from build123d import *

# Parameters (mm, degrees)
SKETCH2_W           = 43.5
SKETCH2_H           = 43.5
BOSS_EXTRUDE1_DEPTH = 5
SKETCH4_W           = 23
SKETCH4_H           = 16
BOSS_EXTRUDE2_DEPTH = 26
SKETCH5_W           = 6
SKETCH5_H           = 10
SKETCH5_W_2         = 12
SKETCH5_H_2         = 6
BOSS_EXTRUDE3_DEPTH = 10
SKETCH6_R           = 2.5
CUT_EXTRUDE1_DEPTH  = 41.275612969


with BuildPart() as part:
    # Sketch2 → Boss-Extrude1 (new body)
    with BuildSketch(Plane(origin=(0, 0, 0), x_dir=(1, 0, 0), z_dir=(0, 1, 0))):
        Rectangle(SKETCH2_W, SKETCH2_H)
    extrude(amount=BOSS_EXTRUDE1_DEPTH)

    # Sketch4 → Boss-Extrude2 (add)
    with BuildSketch(Plane(origin=(0, 5, 0), x_dir=(1, 0, 0), z_dir=(0, 1, 0))):
        with Locations((0, -13.75)):
            Rectangle(SKETCH4_W, SKETCH4_H)
    extrude(amount=BOSS_EXTRUDE2_DEPTH)

    # Sketch5 → Boss-Extrude3 (add)
    with BuildSketch(Plane(origin=(0, 5, 0), x_dir=(1, 0, 0), z_dir=(0, 1, 0))):
        with Locations((-18.75, 9.331650707)):
            Rectangle(SKETCH5_W, SKETCH5_H)
        with Locations((0.664199044, 18.75)):
            Rectangle(SKETCH5_W_2, SKETCH5_H_2)
        with Locations((18.75, 9.243455857)):
            Rectangle(SKETCH5_W, SKETCH5_H)
    extrude(amount=BOSS_EXTRUDE3_DEPTH)

    # Sketch6 → Cut-Extrude1 (cut, through all)
    with BuildSketch(Plane(origin=(0, 5, 0), x_dir=(1, 0, 0), z_dir=(0, 1, 0))):
        with Locations(Location((-18.25, 18.25, 0), (0, 0, 270))):
            Circle(SKETCH6_R)
        with Locations(Location((18.124031363, 18.25, 0), (0, 0, 270))):
            Circle(SKETCH6_R)
        with Locations(Location((18.124031363, -18.25, 0), (0, 0, 270))):
            Circle(SKETCH6_R)
        with Locations(Location((-18.25, -18.25, 0), (0, 0, 270))):
            Circle(SKETCH6_R)
    extrude(amount=-CUT_EXTRUDE1_DEPTH, mode=Mode.SUBTRACT)


solid = part.part
Read the model definition and answer for the solid it produces. Units are mm, in the model's axes. A direction names the side the tool comes from. Coordinates: 2 decimals unless noted, no trailing zeros. Loops run counter-clockwise (first coordinate to the right, second up) from the corner with the lowest first, then second, coordinate; pieces in that order, holes last. Notation, with made-up numbers: (-17, 31) -> (16, 31) arc R18 cw to (16, 41) -> close; hole circle Ø9 at (33, 50). An arc over 180 degrees is marked (long way). Answer in a Markdown table with one row per item.
Item 1: A cutting plane is placed at A-A on y = 9.5. Determine the outline of the cut face in (x, z), plus the area to 3 significant figures.
Returned:
| item | result |
|---|---|
| outline | (-21.75, -14.33) -> (-15.75, -14.33) -> (-15.75, -4.33) -> (-21.75, -4.33) -> close; (-11.5, 5.75) -> (11.5, 5.75) -> (11.5, 21.75) -> (-11.5, 21.75) -> close; (-5.34, -21.75) -> (6.66, -21.75) -> (6.66, -15.75) -> (-5.34, -15.75) -> close; (15.75, -14.24) -> (21.75, -14.24) -> (21.75, -4.24) -> (15.75, -4.24) -> close |
| area | 560 mm^2 |
Item 2: Straight lines are drawn through the part: line 1 along X through (y, z) = (1.15, 18.25); line 2 along Z through (x, y) = (16, 3); line 3 along X through (y, z) = (12, 7). For each, find the intervals that lie inside material, in ascending order. Write a range as [from, to].
Returned:
| item | result |
|---|---|
| line 1 | x = [-21.75, -20.75], [-15.75, 15.62], [20.62, 21.75] |
| line 2 | z = [-21.75, -19.57], [-16.93, 16.93], [19.57, 21.75] |
| line 3 | x = [-11.5, 11.5] |
Item 3: For a pull along X with two mould halves and no side action, classify faces 1 (the flat face through (-19, 10, -14.332)), 2 (the flat face through (15.75, 10, -9)), 3 (the flat face through (11.5, 18, 14)) as released by +X, released by -X, zero draft, split by the parting line, or undercut.
Returned:
| item | result |
|---|---|
| face 1 | zero draft |
| face 2 | undercut |
| face 3 | released by +X |
Item 4: A cutting plane is placed at D-D on x = -6.5. Determine the outline of the cut face in (y, z), plus the area to 4 significant figures.
Returned:
| item | result |
|---|---|
| outline | (0, -21.75) -> (5, -21.75) -> (5, 5.75) -> (31, 5.75) -> (31, 21.75) -> (0, 21.75) -> close |
| area | 633.5 mm^2 |
Item 5: For faces 4 (the flat face through (-19, 10, -4.332)), 5 (the flat face through (19, 10, -14.243)), 6 (the flat face through (1, 10, -15.75)), 7 (the flat face through (-15.75, 10, -9)), determine the directions among +Z, -Z, +X, -X, +Y, -Y from which every point of the face is accessible in a straight line to the end or side of a thin tool.
Returned:
| item | result |
|---|---|
| face 4 | +Z, -X, +Y |
| face 5 | -Z, +X, +Y |
| face 6 | +X, -X, +Y |
| face 7 | +Z, -Z, +Y |
Item 6: A cutting plane is placed at C-C on x = -18.25. Determine the outline of the cut face in (y, z), plus the area to 4 significant figures.
Returned:
| item | result |
|---|---|
| outline | (0, -21.75) -> (5, -21.75) -> (5, -20.75) -> (0, -20.75) -> close; (0, -15.75) -> (5, -15.75) -> (5, -14.33) -> (15, -14.33) -> (15, -4.33) -> (5, -4.33) -> (5, 15.75) -> (0, 15.75) -> close; (0, 20.75) -> (5, 20.75) -> (5, 21.75) -> (0, 21.75) -> close |
| area | 267.5 mm^2 |
Item 7: Each of these flat-tipped pins is pushed along its axis until it touches: P1, Ø5, axis at x = -17.5, z = -11.5, coming from the +Y side; P2, Ø13, axis at y = 22, z = 10.5, coming from the -X side; P3, Ø1.8, axis at x = -18.5, y = 9.5, coming from the -Z side. Where does it stop, or does it pass through?
Returned:
| item | result |
|---|---|
| P1 | stops at y = 15 |
| P2 | stops at x = -11.5 |
| P3 | stops at z = -14.33 |
Item 8: A cutting plane is placed at B-B on z = 18.25. Determine the outline of the cut face in (x, y), plus the area to 4 significant figures.
Returned:
| item | result |
|---|---|
| outline | (-21.75, 0) -> (-20.75, 0) -> (-20.75, 5) -> (-21.75, 5) -> close; (-15.75, 0) -> (15.62, 0) -> (15.62, 5) -> (11.5, 5) -> (11.5, 31) -> (-11.5, 31) -> (-11.5, 5) -> (-15.75, 5) -> close; (20.62, 0) -> (21.75, 0) -> (21.75, 5) -> (20.62, 5) -> close |
| area | 765.5 mm^2 |
